Check sheet for the modelled part. Datum: model origin and axes. Units: mm. Face numbers are marked on the shaded views. Round coordinates to 2 decimals unless told otherwise and drop trailing zeros. Loops run counter-clockwise (first coordinate to the right, second up) from the corner with the lowest first, then second, coordinate; pieces in that order, holes last. Notation, with made-up numbers: (75, 60.5) -> (124, 60.5) arc R29 ccw to (124, 98.5) -> close; hole circle Ø9 at (61.25, 37). An arc over 180 degrees is marked (long way). Return JSON: item names as keys, results as strings.
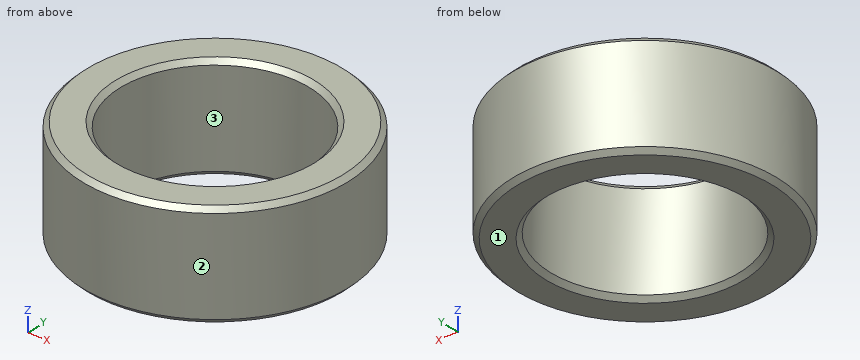
from build123d import *

# Parameters (mm, degrees)
BK_COLLAR_SKETCH_R     = 7
BK_COLLAR_SKETCH_R_2   = 5
BK_COLLAR_DEPTH        = 5.5
BK_COLLAR_CHAMFER_SIZE = 0.25


with BuildPart() as part:
    # BK Collar Sketch → BK Collar (new body)
    with BuildSketch(Plane.XY):
        Circle(BK_COLLAR_SKETCH_R)
        Circle(BK_COLLAR_SKETCH_R_2, mode=Mode.SUBTRACT)
    extrude(amount=BK_COLLAR_DEPTH)

    # BK Collar Chamfer
    bk_collar_chamfer_edges = [part.edges().sort_by_distance(p)[0] for p in [
        (-7, 0, 0),
        (-7, 0, 5.5),
        (-5, 0, 0),
        (-5, 0, 5.5),
    ]]
    chamfer(bk_collar_chamfer_edges, length=BK_COLLAR_CHAMFER_SIZE)


solid = part.part
Q1. Section check A-A (x = 0). Record the boundary of the cut face in (y, z).
Results list:
{"outline": "(-7, 0.25) -> (-6.75, 0) -> (-5.25, 0) -> (-5, 0.25) -> (-5, 5.25) -> (-5.25, 5.5) -> (-6.75, 5.5) -> (-7, 5.25) -> close; (5, 0.25) -> (5.25, 0) -> (6.75, 0) -> (7, 0.25) -> (7, 5.25) -> (6.75, 5.5) -> (5.25, 5.5) -> (5, 5.25) -> close"}
Q2. Draft check along X on the marked faces 1, 2 and 3. Enter one of: released by +X, released by -X, zero draft, split by the parting line, or undercut.
Results list:
{"face 1": "zero draft", "face 2": "split by the parting line", "face 3": "undercut"}
Q3. Go/stop test with flat-tipped pins: pin 1 (6 mm diameter, centred on x = 1.5, y = -2.5, fed in from -Z); pin 2 (1 mm diameter, centred on y = -2, z = 1.5, fed in from -X); pin 3 (1 mm diameter, centred on y = 5, z = 1, fed in from +X); pin 4 (1.5 mm diameter, centred on x = 4, z = 5, fed in from +Y). Record where each tip stops, or that it passes through.
Results list:
{"pin 1": "z = 0", "pin 2": "x = -6.84", "pin 3": "x = 5.36", "pin 4": "y = 6.2"}
Q4. Section check C-C (z = 1.4). Record the boundary of the cut face in (x, y), then the cut area to 3 significant figures.
Results list:
{"outline": "circle Ø14 at (0, 0); hole circle Ø10 at (0, 0)", "area": "75.4 mm^2"}
Q5. Material ranges on line 1 (Y direction, x = 0, z = 3.4); line 2 (Y direction, x = 2.25, z = 4.5); line 3 (X direction, y = -2.75, z = 4.4), recorded low to high.
Results list:
{"line 1": "-7 to -5, 5 to 7", "line 2": "-6.63 to -4.47, 4.47 to 6.63", "line 3": "-6.44 to -4.18, 4.18 to 6.44"}
